CAD build for the part. Positions are in the model's coordinates, mm. Face numbers are marked on the shaded views. A direction names the side the tool comes from. Give positions to 0.01 mm unless a question says otherwise; leave off trailing zeros. Order: outer loops, then holes, each group sorted by start corner. A loop starts at its lowest first (then second) coordinate and runs counter-clockwise, first axis right, second up. Notation, with made-up numbers: M 0,54.25 L 10,54.25 A29 cw 10,83.25 Z; hole C -9,-29 d7. An arc over 180 degrees is marked long. Put each result on its own line as item: value. Start each with the question number.
1) Drill centre lines: line 1 (Y direction, x = -15.5, z = 38.5); line 2 (Z direction, x = 14.5, y = 16); line 3 (Y direction, x = 0, z = 57). Where is each one in solid material? Low to high. Write a range as [from, to].
2) Tool access for the marked faces 1 and 2: list every direction of +Z, -Z, +X, -X, +Y, -Y with a clear straight run to the whole face (end or side of a thin tool).
3) Pin check, flat tips, straight feed: pin 1 (12 mm diameter, centred on x = 15, y = 16, fed in from +Z); pin 2 (1 mm diameter, centred on x = 2, z = 53, fed in from -Y); pin 3 (2.5 mm diameter, centred on x = -15.5, y = 15.5, fed in from +Z). Stop position of each tip, or through.
4) Cut at A-A (x = 15.5). Write the cut outline in (y, z).
5) Cut at C-C (y = -9). Write the cut outline in (x, z), and give its area (3 significant figures).
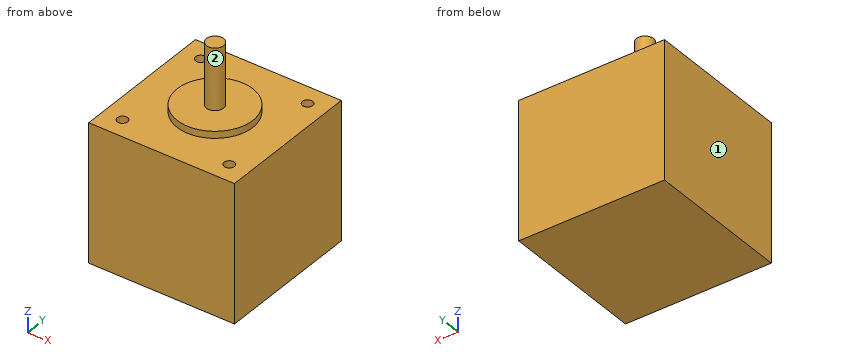
```python
from build123d import *

# Parameters (mm, degrees)
SKETCH_1_W          = 42.3
SKETCH_1_H          = 42.3
EXTRUDE_1533_DEPTH  = 40
SKETCH_2_R          = 2.5
EXTRUDE_1588_DEPTH  = 59.8
SKETCH_3_R          = 11
EXTRUDE_1635_DEPTH  = 42
CUT_EXTRUDE_START   = 40
SKETCH_5_R          = 1.5
CUT_EXTRUDE_3_DEPTH = 4.5


with BuildPart() as part:
    # Эскиз1 → Extrude 1533 (new body)
    with BuildSketch(Plane.XY):
        Rectangle(SKETCH_1_W, SKETCH_1_H)
    extrude(amount=EXTRUDE_1533_DEPTH)

    # Эскиз2 → Extrude 1588 (add)
    with BuildSketch(Plane.XY):
        with Locations(Location((0, 0, 0), (0, 0, 180))):
            Circle(SKETCH_2_R)
    extrude(amount=EXTRUDE_1588_DEPTH)

    # Эскиз3 → Extrude 1635 (add)
    with BuildSketch(Plane.XY):
        with Locations(Location((0, 0, 0), (0, 0, 180))):
            Circle(SKETCH_3_R)
    extrude(amount=EXTRUDE_1635_DEPTH)

    # Эскиз5 → Крепеж_М3_ПРЕДВ (cut)
    with BuildSketch(Plane.XY.offset(CUT_EXTRUDE_START)):
        with Locations((-15.5, -15.5)):
            Circle(SKETCH_5_R)
        with Locations((-15.5, 15.5)):
            Circle(SKETCH_5_R)
        with Locations((15.5, -15.5)):
            Circle(SKETCH_5_R)
        with Locations((15.5, 15.5)):
            Circle(SKETCH_5_R)
    extrude(amount=-CUT_EXTRUDE_3_DEPTH, mode=Mode.SUBTRACT)


solid = part.part
```
Solution:
1. line 1: [-21.15, -17], [-14, 14], [17, 21.15]
1. line 2: [0, 35.5]
1. line 3: [-2.5, 2.5]
2. face 1: +Z, -Z, -X, +Y, -Y
2. face 2: +Z
3. pin 1: z = 40
3. pin 2: y = -2
3. pin 3: z = 35.5
4. outline: M -21.15,0 L 21.15,0 L 21.15,40 L 17,40 L 17,35.5 L 14,35.5 L 14,40 L -14,40 L -14,35.5 L -17,35.5 L -17,40 L -21.15,40 Z
5. outline: M -21.15,0 L 21.15,0 L 21.15,40 L 6.32,40 L 6.32,42 L -6.32,42 L -6.32,40 L -21.15,40 Z
5. area: 1,720 mm²
